Autodesk Inventor part; units mm, degrees
ref_plane "YZ Plane" through (0, 0, 0) normal (1, 0, 0) x (0, 1, 0)
ref_plane "XZ Plane" through (0, 0, 0) normal (0, 1, 0) x (-1, 0, 0)
ref_plane "XY Plane" through (0, 0, 0) normal (0, 0, 1) x (1, 0, 0)
sketch "Sketch1" plane through (0, 0, 0) normal (0, 0, 1) x (1, 0, 0)
  line L0 (-6, 6) -> (6, 6)
  line L1 (6, 6) -> (6, -6)
  line L2 (6, -6) -> (-6, -6)
  line L3 (-6, -6) -> (-6, 6)
  line L4 (-6, 6) -> (6, -6) construction
  line L5 (6, 6) -> (-6, -6) construction
  point P0 (0, 0)
  dimension "d0" = 12
  dimension "d1" = 12
extrude "Extrusion1" add sketch "Sketch1" along normal blind 2
sketch "Sketch2" plane through (0, 0, 0) normal (1, 0, 0) x (0, 1, 0)
  arc A0 (4, 0) -> (-4, 0) centre (0, 0) ccw
  line L0 (-6, 0) -> (6, 0)
  dimension "d4" = 8
sketch "Sketch3" plane through (0, 0, 0) normal (0, 0, -1) x (-1, 0, 0)
  circle A0 centre (0, -4) radius 1
  line L0 (0, 4) -> (0, -4)
  point P0 (0, 0)
  dimension "d5" = 2
sweep "Sweep1" add profiles "Sketch3" path "Sketch2" path curves A0
properties part number "pad"
Geometry check sheet. Reference: the model listing, model coordinates, mm. Coordinates: 2 decimals unless noted, no trailing zeros. Loops run counter-clockwise (first coordinate to the right, second up) from the corner with the lowest first, then second, coordinate; pieces in that order, holes last. Notation, with made-up numbers: (13, -35.75) - (69, -35.75) arc R22 ccw to (69, -3.75) - close; hole circle Ø2 at (-15.5, 47). An arc over 180 degrees is marked (long way). Use one line per item in the form item = value. Start each with the question number.
Item 1: Thickness scan on probe 1 along Z at (x, y) = (2.5, 2); probe 2 along Z at (x, y) = (0, -1.25); probe 3 along X at (y, z) = (-2.5, 4.15). Record the ranges inside material, lowest first.
Item 2: Section check A-A, the plane y = 5.25. Enter the section's corners in (x, z).
Item 3: Gauge pin test, flat end, axial feed: pin 1 (6 mm diameter, centred on x = -2, y = -4, fed in from -Z). Record the tip position at first contact, or that the pin passes through.
Computed:
q1.probe_1 = 0 to 2
q1.probe_2 = 0 to 2, 2.73 to 4.84
q1.probe_3 = -0.54 to 0.54
q2.outline = (-6, 0) - (6, 0) - (6, 2) - (-6, 2) - close
q3.pin_1 = 0
